The model under review builds one solid part; all positions refer to its coordinate system, in mm. Face numbers are marked on the shaded views. Give positions to 0.01 mm unless a question says otherwise; leave off trailing zeros. Loops run counter-clockwise (first coordinate to the right, second up) from the corner with the lowest first, then second, coordinate; pieces in that order, holes last. Notation, with made-up numbers: M 31,-2 L 52,-2 A6 cw 52,4 Z; hole C -23.75,-2 d3. An arc over 180 degrees is marked long. One line per item, written item: value. Start each with the question number.
Q1. We need section D-D on z = 10. Write out the cut boundary in (x, y), plus the area to 3 significant figures.
Q2. Mouldability with a two-part tool opening along Z and no side actions: class the marked faces 1, 2 and 3 as released by +Z, released by -Z, zero draft, split by the parting line, or undercut.
Q3. We need section A-A on x = 1.5. Write out the cut boundary in (y, z).
Q4. We need section B-B on z = -7.5. Write out the cut boundary in (x, y).
Q5. For pin 1 (5 mm diameter, centred on y = -0.5, z = -2.5, fed in from +X); pin 2 (1.5 mm diameter, centred on x = 1, y = 11, fed in from +Z); pin 3 (1 mm diameter, centred on x = 1.5, z = -1, fed in from +Y); pin 4 (0.9 mm diameter, centred on x = 1.5, y = -5, fed in from -Z), all flat-tipped, find the tip position at first contact; note any pin that passes through.
Q6. To check wall thickness, follow line 1 along Y through (x, z) = (1.55, 2); line 2 along Z through (x, y) = (0.4, -7.75); line 3 along Y through (x, z) = (1.7, 4). State the ranges of each line that lie inside material, in increasing order. Write a range as from..to.
Autodesk Inventor part; units mm, degrees
ref_plane "YZ Plane" through (0, 0, 0) normal (1, 0, 0) x (0, 1, 0)
ref_plane "XZ Plane" through (0, 0, 0) normal (0, 1, 0) x (-1, 0, 0)
ref_plane "XY Plane" through (0, 0, 0) normal (0, 0, 1) x (1, 0, 0)
sketch "Boceto1" plane through (0, 0, 0) normal (1, 0, 0) x (0, 1, 0)
  circle A0 centre (0, 0) radius 2.5
  line L0 (2.5, 0) -> (2.5, 10.6639)
  line L1 (2.5, 2.5) -> (-7.5, 2.5)
  line L2 (-7.5, 2.5) -> (-9.5, 2.5)
  line L3 (-9.5, 2.5) -> (-9.5, 4.5)
  line L4 (-9.5, 4.5) -> (2.5, 4.5)
  line L5 (0, 0) -> (-4.5773, -4.5773)
  line L6 (0, 0) -> (6.4732, 0) construction
  circle A1 centre (0, 0) radius 2.5
  line L7 (0, 2.5) -> (10.6639, 2.5)
  line L8 (2.5, 2.5) -> (2.5, -7.5)
  line L9 (2.5, -7.5) -> (2.5, -9.5)
  line L10 (2.5, -9.5) -> (4.5, -9.5)
  line L11 (4.5, -9.5) -> (4.5, 2.5)
  line L12 (2.5, 4.5) -> (4.5, 4.5)
  line L13 (4.5, 4.5) -> (4.5, 2.5)
  point P0 (0, 2.5)
  dimension "d0" = 5
  dimension "d1" = 10
  dimension "d2" = 2
  dimension "d3" = 2
  dimension "d4" = 135
extrude "Extrusión1" add sketch "Boceto1" along normal blind 3 contours A0 L1 L0 | L0 L7 L11 L10 L9 L8 | L1 L2 L3 L4 L0 | L0 L12 L13 L7
sketch "Boceto2" plane through (3, 0, 0) normal (1, 0, 0) x (0, 0, -1)
  line L0 (-4.5, 4.5) -> (-4.5, -9.5)
  line L1 (-2.5, -9.5) -> (-2.5, 0)
  arc A0 (0, 2.5) -> (-2.5, 0) centre (0, 0) ccw
  line L2 (0, 2.5) -> (9.5, 2.5)
  line L3 (9.5, 2.5) -> (9.5, 4.5)
  line L4 (9.5, 4.5) -> (-4.5, 4.5)
  line L5 (-4.5, 4.5) -> (-4.5, -9.5)
  line L6 (-4.5, -9.5) -> (-2.5, -9.5)
  line L7 (9.5, 2.5) -> (9.5, 4.5)
  line L8 (9.5, 4.5) -> (16.7965, 4.5)
  line L9 (16.7965, 2.5) -> (9.5, 2.5)
  line L10 (9.5, 2.5) -> (16.7965, 2.5)
  line L11 (16.7965, 4.5) -> (16.7965, 2.5)
  circle A1 centre (-4.5, 4.5) radius 14
extrude "Extrusión2" add sketch "Boceto2" against normal blind 3 contours L0 A1 L4
sketch "Boceto3" plane through (0, 2.5, -9.5) normal (0, -1, 0) x (1, 0, 0)
  line L0 (0, 0) -> (3, 0)
  line L1 (1.5, 0) -> (1.5, 2)
  circle A0 centre (1.5, 2) radius 1.35
  point P0 (0, 9.5)
  dimension "d9" = 2
  dimension "d10" = 2.7
extrude "Extrusión3" add sketch "Boceto3" along normal blind 1
fillet "Empalme1" radius 0.2 1 edges at (0.15, 1.5, -7.5)
sketch "Boceto4" plane through (0, -9.5, 2.5) normal (0, 0, -1) x (-1, 0, 0)
  line L0 (0, 0) -> (-3, 0)
  line L1 (-1.5, 0) -> (-1.5, 2)
  circle A0 centre (-1.5, 2) radius 1.35
  point P0 (0, 9.5)
  dimension "d14" = 2
  dimension "d15" = 2.7
extrude "Extrusión4" add sketch "Boceto4" along normal blind 1
fillet "Empalme2" radius 0.2 1 edges at (2.85, -7.5, 1.5)
properties part number "oso"
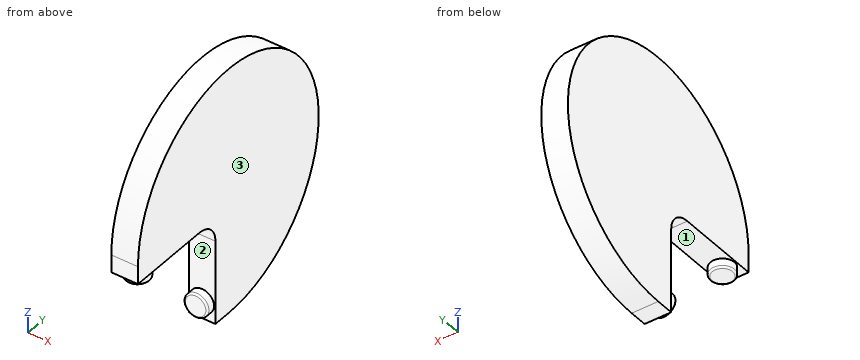
Solved:
1. outline: M 0,-8.37 L 3,-8.37 L 3,17.37 L 0,17.37 Z
1. area: 77.2 mm2
2. face 1: released by -Z
2. face 2: undercut
2. face 3: zero draft
3. outline: M -9.5,2.5 L -8.85,2.5 L -8.85,1.7 A0.2 ccw -8.65,1.5 L -6.35,1.5 A0.2 ccw -6.15,1.7 L -6.15,2.5 L 0,2.5 A2.5 cw 2.5,0 L 2.5,-6.15 L 1.7,-6.15 A0.2 ccw 1.5,-6.35 L 1.5,-8.65 A0.2 ccw 1.7,-8.85 L 2.5,-8.85 L 2.5,-9.5 L 4.5,-9.5 A14 ccw long -9.5,4.5 Z
4. outline: M 0,2.5 L 0.15,2.5 L 0.15,1.7 A0.2 ccw 0.35,1.5 L 2.65,1.5 A0.2 ccw 2.85,1.7 L 2.85,2.5 L 3,2.5 L 3,11.71 L 0,11.71 Z
5. pin 1: through
5. pin 2: z = 17.26
5. pin 3: y = 17.58
5. pin 4: z = 2.5
6. line 1: -8.85..-6.15, 1.5..18.27
6. line 2: 1.5..11.28
6. line 3: -9.5..18.49
